```python
from build123d import *

# Parameters (mm, degrees)
SKETCH1_R           = 3.175
BOSS_EXTRUDE1_DEPTH = 0.508
CUT_REVOLVE1_ANGLE  = 180


with BuildPart() as part:
    # Sketch1 → Boss-Extrude1 (new body)
    with BuildSketch(Plane(origin=(0, 0, 0), x_dir=(1, 0, 0), z_dir=(0, 1, 0))):
        with Locations(Location((0, 0, 0), (0, 0, 270))):
            Circle(SKETCH1_R)
    extrude(amount=BOSS_EXTRUDE1_DEPTH)

    # Sketch2 → Cut-Revolve1 (revolve, cut)
    with BuildSketch(Plane(origin=(0, 0.508, 0), x_dir=(1, 0, 0), z_dir=(0, 1, 0))):
        Polygon((-2.556490895, -1.882811542), (2.556490895, 1.882811542), (2.571471578, 1.862299364), (-2.541346594, -1.903203218), align=None)
    revolve(axis=Axis((-2.556490895, 0.508, 1.882811542), (0.8051939826990212, 0, -0.5930115093531394)), revolution_arc=CUT_REVOLVE1_ANGLE, mode=Mode.SUBTRACT)


solid = part.part
```
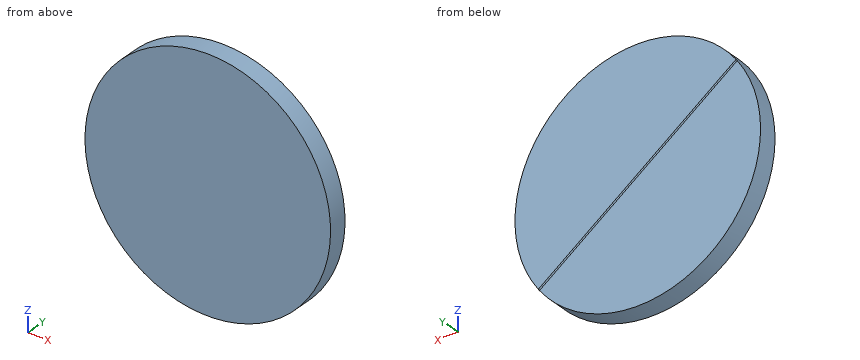
Read the model definition and answer for the solid it produces. Units are mm, in the model's axes. Coordinates: 2 decimals unless noted, no trailing zeros. Loops run counter-clockwise (first coordinate to the right, second up) from the corner with the lowest first, then second, coordinate; pieces in that order, holes last.
(1) The part is cut by section C-C (x = 2.75). Determine the outline of the cut face in (y, z).
Solution:
outline: (0, -1.59) - (0.51, -1.59) - (0.51, 1.59) - (0, 1.59) - close
(2) The part is cut by section B-B (z = 2.5). Determine the outline of the cut face in (x, y).
Solution:
outline: (-1.96, 0) - (1.96, 0) - (1.96, 0.51) - (-1.96, 0.51) - close
(3) The part is cut by section A-A (y = 0.35). Determine the outline of the cut face in (x, z) (3 decimals), and give its area (3 significant figures).
Solution:
outline: circle Ø6.35 at (0, 0)
area: 31.7 mm2
(4) Consider line 1 along X through (y, z) = (0.4, 2.5); line 2 along Z through (x, y) = (-0.5, 0.05); line 3 along Z through (x, y) = (-0.25, 0.35). Determine where each line is inside the solid, lowest interval first.
Solution:
line 1: x = -1.96 to 1.96
line 2: z = -3.14 to 3.14
line 3: z = -3.17 to 3.17
